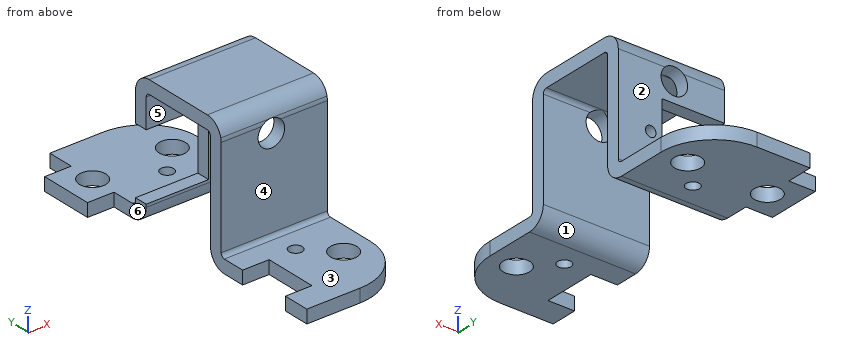
from build123d import *

# Parameters (mm, degrees)
SKETCH1_W           = 40
SKETCH1_H           = 60
SKETCH1_R           = 1.25
BASE_FLANGE1_DEPTH  = 2.5
SKETCH15_R          = 1
CUT_EXTRUDE3_DEPTH  = 10
JOG3_START          = -2.5
JOG3_OUTLINE_W      = 40
JOG3_OUTLINE_H      = 58.294687966
JOG3_OUTLINE_R      = 1
JOG3_OUTLINE_R_2    = 1.25
JOG3_DEPTH          = 2.5
JOG3_2_OUTLINE_W    = 40
JOG3_2_OUTLINE_H    = 1.705312034
JOG3_2_DEPTH        = 0.332528284
JOG3_START_2        = 19.2634
JOG3_3_OUTLINE_W    = 40
JOG3_3_OUTLINE_H    = 40
JOG3_3_OUTLINE_R    = 1
JOG3_3_OUTLINE_R_2  = 1.25
JOG3_3_DEPTH        = 3.2366
JOG3_4_OUTLINE_W    = 40
JOG3_4_OUTLINE_H    = 20.794687966
JOG3_4_OUTLINE_R    = 1.25
JOG3_4_DEPTH        = 3.2366
JOG3_5_OUTLINE_W    = 40
JOG3_5_OUTLINE_H    = 2.5
JOG3_5_DEPTH        = 20
JOG3_START_3        = 20
JOG3_6_OUTLINE_R    = 1.25
JOG3_6_OUTLINE_R_2  = 1
JOG3_6_DEPTH        = 2.5
JOG3_START_4        = -20
JOG3_7_DEPTH        = 40
JOG4_START          = -20
JOG4_DEPTH          = 40
JOG4_2_DEPTH        = 40
JOG4_START_2        = -3
JOG4_3_OUTLINE_R    = 1.25
JOG4_3_DEPTH        = 4
FILLET1_R           = 10
SKETCH18_R          = 2.5
BOSS_EXTRUDE1_DEPTH = 2.5
SKETCH19_R          = 1
SKETCH19_W          = 23.5
SKETCH19_H          = 12.5
CUT_EXTRUDE4_DEPTH  = 2.5
SKETCH20_R          = 2.5
CUT_EXTRUDE6_DEPTH  = 10
SKETCH23_R          = 2.5
CUT_EXTRUDE7_DEPTH  = 51.062460986
SKETCH24_R          = 5
CUT_EXTRUDE8_DEPTH  = 1.25
SKETCH26_R          = 2.5
CUT_EXTRUDE12_DEPTH = 51.062460987
SKETCH27_W          = 20
SKETCH27_H          = 13.5268
CUT_EXTRUDE13_DEPTH = 61.042487703


with BuildPart() as part:
    # Base-Flange1: sheet metal written as solids
    # Sketch1 → Base-Flange1 (new body)
    with BuildSketch(Plane.XY):
        Rectangle(SKETCH1_W, SKETCH1_H)
        with Locations((10, 15)):
            Circle(SKETCH1_R, mode=Mode.SUBTRACT)
        with Locations(Location((10, -15, 0), (0, 0, 180))):
            Circle(SKETCH1_R, mode=Mode.SUBTRACT)
        with Locations((-10, -15)):
            Circle(SKETCH1_R, mode=Mode.SUBTRACT)
        with Locations(Location((-10, 15, 0), (0, 0, 180))):
            Circle(SKETCH1_R, mode=Mode.SUBTRACT)
    extrude(amount=-BASE_FLANGE1_DEPTH)

    # Sketch15 → Cut-Extrude3 (cut)
    with BuildSketch(Plane.XY):
        with Locations((12, 0)):
            Circle(SKETCH15_R)
        with Locations(Location((-17, 0, 0), (0, 0, 180))):
            Circle(SKETCH15_R)
    extrude(amount=-CUT_EXTRUDE3_DEPTH, mode=Mode.SUBTRACT)

    # Jog3: read off the stored shape, not the designer's step
    # Jog3 outline → Jog3 (cut)
    with BuildSketch(Plane.XY.offset(JOG3_START)):
        with Locations((0, -0.852656017)):
            Rectangle(JOG3_OUTLINE_W, JOG3_OUTLINE_H)
        with Locations((-17, 0)):
            Circle(JOG3_OUTLINE_R, mode=Mode.SUBTRACT)
        with Locations((12, 0)):
            Circle(JOG3_OUTLINE_R, mode=Mode.SUBTRACT)
        with Locations((-10, 15)):
            Circle(JOG3_OUTLINE_R_2, mode=Mode.SUBTRACT)
        with Locations((10, 15)):
            Circle(JOG3_OUTLINE_R_2, mode=Mode.SUBTRACT)
        with Locations((10, -15)):
            Circle(JOG3_OUTLINE_R_2, mode=Mode.SUBTRACT)
        with Locations((-10, -15)):
            Circle(JOG3_OUTLINE_R_2, mode=Mode.SUBTRACT)
    extrude(amount=JOG3_DEPTH, mode=Mode.SUBTRACT)

    # Jog3 2 outline → Jog3 2 (cut)
    with BuildSketch(Plane.XY.offset(JOG3_START)):
        with Locations((0, 29.147343983)):
            Rectangle(JOG3_2_OUTLINE_W, JOG3_2_OUTLINE_H)
    extrude(amount=JOG3_2_DEPTH, mode=Mode.SUBTRACT)

    # Jog3 4 outline → Jog3 4 (add)
    with BuildSketch(Plane.XY.offset(JOG3_START)):
        with Locations((0, 40.397343983)):
            Rectangle(JOG3_4_OUTLINE_W, JOG3_4_OUTLINE_H)
        with Locations((10, 35.794687966)):
            Circle(JOG3_4_OUTLINE_R, mode=Mode.SUBTRACT)
        with Locations((-10, 35.794687966)):
            Circle(JOG3_4_OUTLINE_R, mode=Mode.SUBTRACT)
    extrude(amount=JOG3_4_DEPTH)



with BuildPart() as body_2:
    # Jog3 3 outline → Jog3 3 (new body)
    with BuildSketch(Plane.XY.offset(JOG3_START_2)):
        with Locations((0, 10.794687966)):
            Rectangle(JOG3_3_OUTLINE_W, JOG3_3_OUTLINE_H)
        with Locations((12, 20.794687966)):
            Circle(JOG3_3_OUTLINE_R, mode=Mode.SUBTRACT)
        with Locations((-17, 0)):
            Circle(JOG3_3_OUTLINE_R, mode=Mode.SUBTRACT)
        with Locations((-10, 5.794687966)):
            Circle(JOG3_3_OUTLINE_R_2, mode=Mode.SUBTRACT)
        with Locations((12, 0)):
            Circle(JOG3_3_OUTLINE_R, mode=Mode.SUBTRACT)
        with Locations((10, 5.794687966)):
            Circle(JOG3_3_OUTLINE_R_2, mode=Mode.SUBTRACT)
        with Locations((-17, 20.794687966)):
            Circle(JOG3_3_OUTLINE_R, mode=Mode.SUBTRACT)
        with Locations((-10, 15)):
            Circle(JOG3_3_OUTLINE_R_2, mode=Mode.SUBTRACT)
        with Locations((10, 15)):
            Circle(JOG3_3_OUTLINE_R_2, mode=Mode.SUBTRACT)
    extrude(amount=JOG3_3_DEPTH)


with BuildPart() as part_1:
    add(part.part)

    add(body_2.part)  # Jog3 5 merges body 2
    # Jog3 5 outline → Jog3 5 (add)
    with BuildSketch(Plane.XY):
        with Locations((0, 29.544687966)):
            Rectangle(JOG3_5_OUTLINE_W, JOG3_5_OUTLINE_H)
    extrude(amount=JOG3_5_DEPTH)

    # Jog3 6 outline → Jog3 6 (add)
    with BuildSketch(Plane.XY.offset(JOG3_START_3)):
        with Locations((10, 15)):
            Circle(JOG3_6_OUTLINE_R)
        with Locations((-10, 15)):
            Circle(JOG3_6_OUTLINE_R)
        with Locations((12, 0)):
            Circle(JOG3_6_OUTLINE_R_2)
        with Locations((-17, 0)):
            Circle(JOG3_6_OUTLINE_R_2)
    extrude(amount=JOG3_6_DEPTH)

    # Jog3 7 outline → Jog3 7 (cut)
    with BuildSketch(Plane.YZ.offset(JOG3_START_4)):
        with BuildLine():
            ThreePointArc((28.294687966, 19.2634), (28.078942821, 19.784254855), (27.558087966, 20))
            Line((27.558087966, 20), (-9.205312034, 20))
            Line((-9.205312034, 20), (-9.205312034, 19.2634))
            Line((-9.205312034, 19.2634), (28.294687966, 19.2634))
        make_face()
        with BuildLine():
            ThreePointArc((31.531287966, -2.5), (29.242666158, -1.552021808), (28.294687966, 0.7366))
            Line((28.294687966, 0.7366), (28.294687966, -2.167471716))
            Line((28.294687966, -2.167471716), (30, -2.167471716))
            Line((30, -2.167471716), (30, -2.5))
            Line((30, -2.5), (31.531287966, -2.5))
        make_face()
        with BuildLine():
            Line((31.531287966, 0), (50.794687966, 0))
            Line((50.794687966, 0), (50.794687966, 0.7366))
            Line((50.794687966, 0.7366), (30.794687966, 0.7366))
            ThreePointArc((30.794687966, 0.7366), (31.010433111, 0.215745145), (31.531287966, 0))
        make_face()
        with BuildLine():
            Line((30.794687966, 22.5), (27.558087966, 22.5))
            ThreePointArc((27.558087966, 22.5), (29.846709774, 21.552021808), (30.794687966, 19.2634))
            Line((30.794687966, 19.2634), (30.794687966, 22.5))
        make_face()
    extrude(amount=JOG3_7_DEPTH, mode=Mode.SUBTRACT)

    # Jog4: read off the stored shape, not the designer's step
    # Jog4 outline → Jog4 (cut)
    with BuildSketch(Plane.YZ.offset(JOG4_START)):
        with BuildLine():
            Line((-9.205312034, 20), (10.87962174, 20))
            ThreePointArc((10.87962174, 20), (12.019882984, 21.799110859), (14.031287966, 22.5))
            Line((14.031287966, 22.5), (-9.205312034, 22.5))
            Line((-9.205312034, 22.5), (-9.205312034, 20))
        make_face()
    extrude(amount=JOG4_DEPTH, mode=Mode.SUBTRACT)

    # Jog4 2 outline → Jog4 2 (add)
    with BuildSketch(Plane.YZ.offset(JOG4_START)):
        with BuildLine():
            Line((-9.205312034, 0), (-9.205312034, -2.5))
            Line((-9.205312034, -2.5), (10.058087966, -2.5))
            ThreePointArc((10.058087966, -2.5), (12.346709774, -1.552021808), (13.294687966, 0.7366))
            Line((13.294687966, 0.7366), (13.294687966, 19.2634))
            ThreePointArc((13.294687966, 19.2634), (13.510433111, 19.784254855), (14.031287966, 20))
            Line((14.031287966, 20), (10.87962174, 20))
            ThreePointArc((10.87962174, 20), (10.81599152, 19.634140241), (10.794687966, 19.2634))
            Line((10.794687966, 19.2634), (10.794687966, 0.7366))
            ThreePointArc((10.794687966, 0.7366), (10.578942821, 0.215745145), (10.058087966, 0))
            Line((10.058087966, 0), (-9.205312034, 0))
        make_face()
    extrude(amount=JOG4_2_DEPTH)

    # Jog4 3 outline → Jog4 3 (cut)
    with BuildSketch(Plane.XY.offset(JOG4_START_2)):
        with Locations((-10, 5.794687966)):
            Circle(JOG4_3_OUTLINE_R)
        with Locations((10, 5.794687966)):
            Circle(JOG4_3_OUTLINE_R)
    extrude(amount=JOG4_3_DEPTH, mode=Mode.SUBTRACT)

    # Fillet1
    fillet1_edges = [part_1.edges().sort_by_distance(p)[0] for p in [
        (20, -9.205312034, -1.25),
        (-20, -9.205312034, -1.25),
        (-20, 50.794687966, -1.25),
        (20, 50.794687966, -1.25),
    ]]
    fillet(fillet1_edges, radius=FILLET1_R)

    # Sketch18 → Boss-Extrude1 (add)
    with BuildSketch(Plane.XY.offset(22.5)):
        with Locations((12, 20.794687966)):
            Circle(SKETCH18_R)
        with Locations((-17, 20.794687966)):
            Circle(SKETCH18_R)
    extrude(amount=-BOSS_EXTRUDE1_DEPTH)

    # Sketch19 → Cut-Extrude4 (cut)
    with BuildSketch(Plane(origin=(0, 30.794687966, 0), x_dir=(1, 0, 0), z_dir=(0, 1, 0))):
        with Locations(Location((13.9, -7.5, 0), (0, 0, 270))):
            Circle(SKETCH19_R)
        with Locations(Location((-13.9, -7.5, 0), (0, 0, 90))):
            Circle(SKETCH19_R)
        with Locations((0, -7.5)):
            Rectangle(SKETCH19_W, SKETCH19_H)
    extrude(amount=-CUT_EXTRUDE4_DEPTH, mode=Mode.SUBTRACT)

    # Sketch20 → Cut-Extrude6 (cut)
    with BuildSketch(Plane.XY):
        with Locations((0, 40.794687966)):
            Circle(SKETCH20_R)
        with Locations(Location((0, 0.794687966, 0), (0, 0, 180))):
            Circle(SKETCH20_R)
        with Locations((15, 0.794687966)):
            Circle(SKETCH20_R)
        with Locations(Location((-15, 0.794687966, 0), (0, 0, 180))):
            Circle(SKETCH20_R)
        with Locations(Location((15, 40.794687966, 0), (0, 0, 180))):
            Circle(SKETCH20_R)
        with Locations((-15, 40.794687966)):
            Circle(SKETCH20_R)
    extrude(amount=-CUT_EXTRUDE6_DEPTH, mode=Mode.SUBTRACT)

    # Sketch23 → Cut-Extrude7 (cut, through all)
    with BuildSketch(Plane(origin=(0, 30.794687966, 0), x_dir=(1, 0, 0), z_dir=(0, 1, 0))):
        with Locations(Location((-5.55, -7.5, 0), (0, 0, 270))):
            Circle(SKETCH23_R)
    extrude(amount=-CUT_EXTRUDE7_DEPTH, mode=Mode.SUBTRACT)

    # Sketch24 → Cut-Extrude8 (cut)
    with BuildSketch(Plane(origin=(0, 13.294687966, 0), x_dir=(1, 0, 0), z_dir=(0, 1, 0))):
        with Locations(Location((-5.55, -7.5, 0), (0, 0, 270))):
            Circle(SKETCH24_R)
    extrude(amount=-CUT_EXTRUDE8_DEPTH, mode=Mode.SUBTRACT)

    # Sketch26 → Cut-Extrude12 (cut, through all)
    with BuildSketch(Plane.XZ.offset(-10.794687966)):
        with Locations(Location((9.45, 17.5, 0), (0, 0, 135.141364755))):
            Circle(SKETCH26_R)
    extrude(amount=-CUT_EXTRUDE12_DEPTH, mode=Mode.SUBTRACT)

    # Sketch27 → Cut-Extrude13 (cut, through all)
    with BuildSketch(Plane.XY.offset(22.5)):
        with Locations((-10, 20.794687966)):
            Rectangle(SKETCH27_W, SKETCH27_H)
        Polygon((0, 45.794687966), (0, 50.794687966), (-20, 50.794687966), (-20, 27.558087966), (0, 27.558087966), (0, 35.794687966), (-5, 35.794687966), (-5, 45.794687966), align=None)
        Polygon((0, 14.031287966), (-20, 14.031287966), (-20, -9.205312034), (0, -9.205312034), (0, -4.205312034), (5, -4.205312034), (5, 5.794687966), (0, 5.794687966), align=None)
    extrude(amount=-CUT_EXTRUDE13_DEPTH, mode=Mode.SUBTRACT)


solid = part_1.part
Input: part model. Units: mm. Frame: model coordinates. Face numbers are marked on the shaded views. A direction names the side the tool comes from. Coordinates: 2 decimals unless noted, no trailing zeros. Loops run counter-clockwise (first coordinate to the right, second up) from the corner with the lowest first, then second, coordinate; pieces in that order, holes last.
(1) Section B-B on z = 17.5. Return the cut outline in (x, y), then the cut area to 3 significant figures.
(2) Set-up query: the marked faces 4, 5 and 6. Return all of +Z, -Z, +X, -X, +Y, -Y with unobstructed straight access to the full face (end or side cutting, diameter ignored); none if empty.
(3) Material intervals for probe 1 along Y at (x, z) = (16.75, 18.25); probe 2 along Z at (x, y) = (9.45, 29.55); probe 3 along Y at (x, z) = (15, -1.1), sorted ascending.
(4) Pull-direction query (Y, two-part tool) for the marked faces 1, 2 and 3; classes: released by +Y, released by -Y, zero draft, split by the parting line, or undercut.
(5) Section D-D on x = 18.75. Return the cut outline in (y, z), then the cut area to 3 significant figures.
(6) First-contact query: pin 1 Ø3 at (y, z) = (33, 0) entering from -X; pin 2 Ø12 at (x, z) = (14.5, 13) entering from +Y; pin 3 Ø11 at (x, y) = (7.5, 20) entering from -Z. Flat tips, straight axial feed; report the tip coordinate or a pass-through.
(7) Section A-A on z = 7.5. Return the cut outline in (x, y).
(8) Section C-C on x = -1.25. Return the cut outline in (y, z).
Data:
1. outline: (0, 10.79) - (6.95, 10.79) - (6.95, 13.29) - (0, 13.29) - close; (0, 28.29) - (6.95, 28.29) - (6.95, 30.79) - (0, 30.79) - close; (11.95, 10.79) - (20, 10.79) - (20, 13.29) - (11.95, 13.29) - close; (11.95, 28.29) - (20, 28.29) - (20, 30.79) - (11.95, 30.79) - close
1. area: 75.0 mm2
2. face 4: +Z, +X, -X, -Y
2. face 5: -Z, +X, -X
2. face 6: +Z, -Z, -X, -Y
3. probe 1: y = 10.79 to 13.29, 28.29 to 30.79
3. probe 2: z = -1.82 to 1.25, 13.75 to 15, 20 to 21.81
3. probe 3: y = -7.87 to -1.71, 3.29 to 12.72, 28.87 to 38.29, 43.29 to 49.45
4. face 1: undercut
4. face 2: released by +Y
4. face 3: zero draft
5. outline: (-4.05, -2.5) - (10.06, -2.5) arc R3.24 ccw to (13.29, 0.74) - (13.29, 19.26) arc R0.74 cw to (14.03, 20) - (27.56, 20) arc R0.74 cw to (28.29, 19.26) - (28.29, 0.74) arc R3.24 ccw to (31.53, -2.5) - (45.64, -2.5) - (45.64, 0) - (31.53, 0) arc R0.74 cw to (30.79, 0.74) - (30.79, 19.26) arc R3.24 ccw to (27.56, 22.5) - (14.03, 22.5) arc R3.24 ccw to (10.79, 19.26) - (10.79, 0.74) arc R0.74 cw to (10.06, 0) - (-4.05, 0) - close
5. area: 228 mm2
6. pin 1: stops at x = 0
6. pin 2: stops at y = 30.79
6. pin 3: stops at z = 20
7. outline: (0, 10.79) - (20, 10.79) - (20, 13.29) - (0, 13.29) - close; (11.75, 28.29) - (12.9, 28.29) - (12.9, 30.79) - (11.75, 30.79) - close; (14.9, 28.29) - (20, 28.29) - (20, 30.79) - (14.9, 30.79) - close
8. outline: (35.79, -2.5) - (38.63, -2.5) - (38.63, 0) - (35.79, 0) - close; (42.96, -2.5) - (45.79, -2.5) - (45.79, 0) - (42.96, 0) - close
